Can you work these out from the model? Positions are in its coordinate system, mm. A direction names the side the tool comes from. Coordinates: 2 decimals unless noted, no trailing zeros. Write each loop counter-clockwise with the first axis right and the second up, starting at its lowest first coordinate (ties: lowest second). Pieces come first, ordered by that corner, then holes. Notation, with made-up numbers: M 10.5,8 L 60.5,8 A21 ccw 60.5,46 Z; hole C 72.5,-29 d9. An arc over 180 degrees is marked long. Answer as a JSON object with one key per item and string values. Group by question number.
from build123d import *

# Parameters (mm, degrees)
F0_W     = 234.95
F0_H     = 914.4
F1_DEPTH = 19.05
F2_W     = 133.35
F2_H     = 76.2
F3_DEPTH = 19.05
F4_R     = 50.8


with BuildPart() as f1:
    # F0 (on Top) → F1 (new body)
    with BuildSketch(Plane.XY):
        with Locations((117.475, -457.2)):
            Rectangle(F0_W, F0_H)
    extrude(amount=F1_DEPTH)

    # F2 (on face) → F3 (cut)
    with BuildSketch(Plane.XY.offset(19.05)):
        with Locations((117.475, -876.3)):
            Rectangle(F2_W, F2_H)
    extrude(amount=-F3_DEPTH, mode=Mode.SUBTRACT)

    # F4
    f4_edges = [f1.edges().sort_by_distance(p)[0] for p in [
        (50.8, -838.2, 9.525),
        (184.15, -838.2, 9.525),
    ]]
    fillet(f4_edges, radius=F4_R)


solid = f1.part
Q1. We'd pull the mould along X, two halves only. Please class faces 3 (the flat face through (0, -464, 9)), 4 (the flat face through (234.95, -464, 9)), 5 (the cylindrical face through (169.664, -853.476, 9.392)), 6 (the flat face through (116, -451, 19.05)): pulls with the +X half, pulls with the -X half, needs draft (parallel to the pull), parting line crosses it, or undercut.
Q2. If we section it at C-C on x = 72.5: List the corners of the cut face in (y, z) for me.
Q3. If we section it at B-B on x = 122.5: List the corners of the cut face in (y, z) for me.
Q4. Will these pins go through, and if not, where does the flat tip stop? pin 1 (1 mm diameter, centred on x = 142.5, z = 10.5, fed in from -Y) (3 decimals); pin 2 (5.5 mm diameter, centred on x = 121, z = 5.5, fed in from -Y).
Q5. On a 3-axis mill with a long thin cutter (end or side, diameter ignored), from which of +Z, -Z, +X, -X, +Y, -Y can I reach the whole of each face in a straight line? I mean faces 1 (the flat face through (117, -838.2, 10)), 2 (the flat face through (116, -451, 0)). Say none if no direction works.
Q6. Please list where these lines run through material, in increasing order: L1, parallel to Y at x = 120, z = 13.75; L2, parallel to Y at x = 75, z = 16.
Q7. If we section it at A-A on z = 5: List the corners of the cut face in (x, y) for me.
Reply:
{
 "1": {"face 3": "pulls with the -X half", "face 4": "pulls with the +X half", "face 5": "undercut", "face 6": "needs draft"},
 "2": {"outline": "M -847.36,0 L 0,0 L 0,19.05 L -847.36,19.05 Z"},
 "3": {"outline": "M -838.2,0 L 0,0 L 0,19.05 L -838.2,19.05 Z"},
 "4": {"pin 1": "y = -839.125", "pin 2": "y = -838.2"},
 "5": {"face 1": "+Z, -Z, -Y", "face 2": "-Z, +X, -X, +Y, -Y"},
 "6": {"L1": "-838.2 to 0", "L2": "-845.72 to 0"},
 "7": {"outline": "M 0,-914.4 L 50.8,-914.4 L 50.8,-889 A50.8 cw 101.6,-838.2 L 133.35,-838.2 A50.8 cw 184.15,-889 L 184.15,-914.4 L 234.95,-914.4 L 234.95,0 L 0,0 Z"}
}
